from build123d import *

# Parameters (mm, degrees)
SCHIZZO2_R                     = 0.75
ESTRUSIONE_ESTRUSIONE1_DEPTH   = 4
TAGLIO_ESTRUSIONE1_START       = 0.5
TAGLIO_ESTRUSIONE1_OUTLINE_R   = 0.75
TAGLIO_ESTRUSIONE1_DEPTH       = 3
TAGLIO_ESTRUSIONE1_START_2     = 1.25
TAGLIO_ESTRUSIONE1_2_OUTLINE_R = 0.75
TAGLIO_ESTRUSIONE1_2_DEPTH     = 1.5
SCHIZZO5_W                     = 7
SCHIZZO5_H                     = 3
TAGLIO_ESTRUSIONE4_DEPTH       = 10
SCHIZZO6_W                     = 4
SCHIZZO6_H                     = 1.5
TAGLIO_ESTRUSIONE5_DEPTH       = 17.747826397


# Read off the part's stored shape, not the designer's step: Taglio-Estrusione1
with BuildPart() as part:
    # Schizzo2 → Estrusione-Estrusione1 (new body)
    with BuildSketch(Plane.XY):
        with BuildLine():
            Line((-1.674960789, 7.009651551), (1.325039211, 7.009651551))
            ThreePointArc((1.325039211, 7.009651551), (2.032145992, 6.716758332), (2.325039211, 6.009651551))
            Line((2.325039211, 6.009651551), (2.325039211, 5.009651551))
            ThreePointArc((2.325039211, 5.009651551), (2.61793243, 4.30254477), (3.325039211, 4.009651551))
            Line((3.325039211, 4.009651551), (4.807645267, 4.009651551))
            ThreePointArc((4.807645267, 4.009651551), (5.267175084, 4.121489209), (5.623919425, 4.431986858))
            Line((5.623919425, 4.431986858), (6.480368598, 5.642199868))
            ThreePointArc((6.480368598, 5.642199868), (7.127920386, 6.050198789), (7.87430745, 5.880809333))
            Line((7.87430745, 5.880809333), (8.967214405, 5.107375855))
            ThreePointArc((8.967214405, 5.107375855), (9.321590916, 4.653454003), (9.366876691, 4.079366068))
            Line((9.366876691, 4.079366068), (8.871648882, 1.793499009))
            ThreePointArc((8.871648882, 1.793499009), (-2.862577448, 0.385742883), (-14.674960789, 0.009651551))
            Line((-14.674960789, 0.009651551), (-14.674960789, 4.009651551))
            Line((-14.674960789, 4.009651551), (-3.674960789, 4.009651551))
            ThreePointArc((-3.674960789, 4.009651551), (-2.967854008, 4.30254477), (-2.674960789, 5.009651551))
            Line((-2.674960789, 5.009651551), (-2.674960789, 6.009651551))
            ThreePointArc((-2.674960789, 6.009651551), (-2.38206757, 6.716758332), (-1.674960789, 7.009651551))
        make_face()
        with Locations((-0.174960789, 5.509651551)):
            Circle(SCHIZZO2_R, mode=Mode.SUBTRACT)
        with Locations((7.577394386, 4.07554752)):
            Circle(SCHIZZO2_R, mode=Mode.SUBTRACT)
    extrude(amount=ESTRUSIONE_ESTRUSIONE1_DEPTH)

    # Taglio-Estrusione1 outline → Taglio-Estrusione1 (cut)
    with BuildSketch(Plane.XY.offset(TAGLIO_ESTRUSIONE1_START)):
        with BuildLine():
            ThreePointArc((-14.674960789, 0.509651551), (-5.658443288, 0.703091506), (3.325039211, 1.498106631))
            Line((3.325039211, 1.498106631), (3.325039211, 4.009651551))
            ThreePointArc((3.325039211, 4.009651551), (2.61793243, 4.30254477), (2.325039211, 5.009651551))
            Line((2.325039211, 5.009651551), (2.325039211, 6.009651551))
            ThreePointArc((2.325039211, 6.009651551), (2.032145992, 6.716758332), (1.325039211, 7.009651551))
            Line((1.325039211, 7.009651551), (-1.674960789, 7.009651551))
            ThreePointArc((-1.674960789, 7.009651551), (-2.38206757, 6.716758332), (-2.674960789, 6.009651551))
            Line((-2.674960789, 6.009651551), (-2.674960789, 5.009651551))
            ThreePointArc((-2.674960789, 5.009651551), (-2.967854008, 4.30254477), (-3.674960789, 4.009651551))
            Line((-3.674960789, 4.009651551), (-14.674960789, 4.009651551))
            Line((-14.674960789, 4.009651551), (-14.674960789, 0.509651551))
        make_face()
        with Locations((-0.174960789, 5.509651551)):
            Circle(TAGLIO_ESTRUSIONE1_OUTLINE_R, mode=Mode.SUBTRACT)
    extrude(amount=TAGLIO_ESTRUSIONE1_DEPTH, mode=Mode.SUBTRACT)

    # Taglio-Estrusione1 2 outline → Taglio-Estrusione1 2 (cut)
    with BuildSketch(Plane.XY.offset(TAGLIO_ESTRUSIONE1_START_2)):
        with BuildLine():
            ThreePointArc((3.325039211, 1.498106631), (6.158824123, 1.87511554), (8.983990596, 2.312044653))
            Line((8.983990596, 2.312044653), (9.366876691, 4.079366068))
            ThreePointArc((9.366876691, 4.079366068), (9.321590916, 4.653454003), (8.967214405, 5.107375855))
            Line((8.967214405, 5.107375855), (7.87430745, 5.880809333))
            ThreePointArc((7.87430745, 5.880809333), (7.127920386, 6.050198789), (6.480368598, 5.642199868))
            Line((6.480368598, 5.642199868), (5.623919425, 4.431986858))
            ThreePointArc((5.623919425, 4.431986858), (5.267175084, 4.121489209), (4.807645267, 4.009651551))
            Line((4.807645267, 4.009651551), (3.325039211, 4.009651551))
            Line((3.325039211, 4.009651551), (3.325039211, 1.498106631))
        make_face()
        with Locations((7.577394386, 4.07554752)):
            Circle(TAGLIO_ESTRUSIONE1_2_OUTLINE_R, mode=Mode.SUBTRACT)
    extrude(amount=TAGLIO_ESTRUSIONE1_2_DEPTH, mode=Mode.SUBTRACT)

    # Schizzo5 → Taglio-Estrusione4 (cut)
    with BuildSketch(Plane(origin=(0, 0, 0), x_dir=(1, 0, 0), z_dir=(0, 1, 0))):
        with Locations((7.3, 0.75)):
            Rectangle(SCHIZZO5_W, SCHIZZO5_H)
        with Locations((7.3, -4.75)):
            Rectangle(SCHIZZO5_W, SCHIZZO5_H)
    extrude(amount=TAGLIO_ESTRUSIONE4_DEPTH, mode=Mode.SUBTRACT)

    # Schizzo6 → Taglio-Estrusione5 (cut, through all)
    with BuildSketch(Plane(origin=(0, 7.009651551, 0), x_dir=(1, 0, 0), z_dir=(0, 1, 0))):
        with Locations((6.983990596, -2)):
            Rectangle(SCHIZZO6_W, SCHIZZO6_H)
    extrude(amount=-TAGLIO_ESTRUSIONE5_DEPTH, mode=Mode.SUBTRACT)


solid = part.part
CAD build for the part. Positions are in the model's coordinates, mm. A direction names the side the tool comes from. Give positions to 0.01 mm unless a question says otherwise; leave off trailing zeros. Order: outer loops, then holes, each group sorted by start corner. A loop starts at its lowest first (then second) coordinate and runs counter-clockwise, first axis right, second up. Notation, with made-up numbers: (-36.5, -29.75) - (19.5, -29.75) arc R13 cw to (19.5, -18.75) - close; hole circle Ø1 at (33, -13). An arc over 180 degrees is marked (long way). Answer in a Markdown table with one row per item.
1. Flat gauge pins, fed straight in: pin 1 (1.5 mm diameter, centred on x = 6.5, y = 2.5, fed in from +Z); pin 2 (0.8 mm diameter, centred on y = 3, z = 1, fed in from -X); pin 3 (0.8 mm diameter, centred on y = 3, z = 4, fed in from +X). Where does each tip first touch, or does it go through?
Data:
| item | result |
|---|---|
| pin 1 | stops at z = 3.25 |
| pin 2 | stops at x = 3.33 |
| pin 3 | stops at x = 3.8 |
2. Tool access for faces 1 (the cylindrical face through (-2.98, 4.29, 0.25)), 2 (the flat face through (4, 4.01, 3)): list every direction of +Z, -Z, +X, -X, +Y, -Y with a clear straight run to the whole face (end or side of a thin tool).
Data:
| item | result |
|---|---|
| face 1 | +Z, -Z, -X, +Y |
| face 2 | +Z, -Z, +Y |
3. Saw through at C-C, the plane z = 1.75. Give the cut face in (x, y).
Data:
| item | result |
|---|---|
| outline | (-14.67, 0.01) arc R135 ccw to (4.98, 1.21) - (4.98, 1.71) arc R135 cw to (-14.67, 0.51) - close |
4. Pull direction Z, two halves, no side cores. Call faces 3 (the flat face through (-5, 3, 4)), 4 (the cylindrical face through (-0.34, 4.78, 3.75)), 5 (the flat face through (-6, 3, 0.5)): pulls with the +Z half, pulls with the -Z half, needs draft (parallel to the pull), parting line crosses it, or undercut.
Data:
| item | result |
|---|---|
| face 3 | pulls with the +Z half |
| face 4 | needs draft |
| face 5 | undercut |
5. Saw through at A-A, the plane y = 2.75. Give the cut face in (x, z).
Data:
| item | result |
|---|---|
| outline | (-14.67, 0) - (3.8, 0) - (3.8, 0.75) - (9.08, 0.75) - (9.08, 1.25) - (3.33, 1.25) - (3.33, 0.5) - (-14.67, 0.5) - close; (-14.67, 3.5) - (3.33, 3.5) - (3.33, 2.75) - (9.08, 2.75) - (9.08, 3.25) - (3.8, 3.25) - (3.8, 4) - (-14.67, 4) - close |
6. Saw through at B-B, the plane x = -8.5. Give the cut face in (y, z).
Data:
| item | result |
|---|---|
| outline | (0.08, 0) - (4.01, 0) - (4.01, 0.5) - (0.58, 0.5) - (0.58, 3.5) - (4.01, 3.5) - (4.01, 4) - (0.08, 4) - close |
7. Probe probe 1 along Z at (x, y) = (6, 4); probe 2 along Z at (x, y) = (0.5, 6.5); probe 3 along Y at (x, z) = (-1.5, 0.25). List the from-to ranges inside material, lowest first. Write a range as [from, to].
Data:
| item | result |
|---|---|
| probe 1 | z = [0.75, 1.25], [2.75, 3.25] |
| probe 2 | z = [0, 0.5], [3.5, 4] |
| probe 3 | y = [0.5, 7.01] |
8. Saw through at D-D, the plane x = -4. Give the cut face in (y, z), plus the area to 3 significant figures.
Data:
| item | result |
|---|---|
| outline | (0.3, 0) - (4.01, 0) - (4.01, 0.5) - (0.8, 0.5) - (0.8, 3.5) - (4.01, 3.5) - (4.01, 4) - (0.3, 4) - close |
| area | 5.21 mm² |
